```python
from build123d import *

# Parameters (mm, degrees)
SKETCH001_R  = 4.5
HOLE_DEPTH   = 25
POCKET_DEPTH = 10


with BuildPart() as part:
    # Sketch → Revolution (revolve)
    with BuildSketch(Plane.XZ):
        Polygon((0, 0), (0, 15), (5.15, 15), (5.15, 4), (7, 4), (7, 0), align=None)
    revolve(axis=Axis((0, 0, 0), (0, 0, 1)))

    # Sketch001 (on Face1 of Revolution) → Hole (cut)
    with BuildSketch(Plane(origin=(0, 0, 15), x_dir=(-1, 0, 0), z_dir=(0, 0, 1))):
        Circle(SKETCH001_R)
    extrude(amount=-HOLE_DEPTH, mode=Mode.SUBTRACT)

    # Sketch002 → Pocket (cut, symmetric)
    with BuildSketch(Plane.XZ):
        Polygon((-1.9, 15), (-1.9, 11), (-5.15, 11), (-5.15, 15), (-5.15, 18.504541), (5.249575, 18.504541), (5.249575, 15), (5.249575, 11), (1.9, 11), (1.9, 15), align=None)
    extrude(amount=POCKET_DEPTH, both=True, mode=Mode.SUBTRACT)


solid = part.part
```
CAD build for the part. Positions are in the model's coordinates, mm. A direction names the side the tool comes from. Round coordinates to 2 decimals unless told otherwise and drop trailing zeros. Order: outer loops, then holes, each group sorted by start corner. A loop starts at its lowest first (then second) coordinate and runs counter-clockwise, first axis right, second up.
Q1. Which spindle directions (+Z, -Z, +X, -X, +Y, -Y) get a long thin tool onto all of the face, cutting with end or side? Do faces 4 (the flat face through (4, 4, 4)), 5 (the flat face through (0, 5, 15)), 6 (the flat face through (5, 0, 11)), 7 (the flat face through (-5, 0, 11)). Say none if no direction does.
Q2. Two-plate mould, pull along X, no slides. Class faces 1 (the flat face through (0, -5, 15)), 2 (the cylindrical face through (4.496, -0.198, 5.938)), 3 (the cylindrical face through (-5.145, 0.226, 8.201)): pulls with the +X half, pulls with the -X half, needs draft (parallel to the pull), parting line crosses it, or undercut.
Q3. Drop flat-ended pins along their axis: pin 1 (1 mm diameter, centred on x = 4, y = 0.5, fed in from +Z); pin 2 (0.6 mm diameter, centred on y = 4.5, z = 13, fed in from -X); pin 3 (6 mm diameter, centred on x = 5.5, y = -1, fed in from -Z); pin 4 (1.5 mm diameter, centred on x = 4, z = 8, fed in from -Y) (3 decimals). Give the stop position or say it passes through.
Q4. Slice it at A-A (z = 11.5). Write the cut outline in (x, y).
Q5. Wall check: L1, parallel to Y at x = 0, z = 9.25; L2, parallel to Y at x = 0, z = 3.5. Give the ranges that are in metal, low to high.
Q6. Slice it at B-B (y = 0). Write the cut outline in (x, z).
Q7. Slice it at D-D (z = 1.75). Write the cut outline in (x, y), and give its area (3 significant figures).
Q8. Slice it at C-C (x = 0). Write the cut outline in (y, z).
Results below:
1. face 4: +Z
1. face 5: +Z, +X, -X, +Y, -Y
1. face 6: +Z, +X, +Y, -Y
1. face 7: +Z, -X, +Y, -Y
2. face 1: needs draft
2. face 2: undercut
2. face 3: parting line crosses it
3. pin 1: stops at z = 11
3. pin 2: stops at x = -1.9
3. pin 3: stops at z = 0
3. pin 4: stops at y = -3.995
4. outline: (-1.9, -4.79) arc R5.15 ccw to (1.9, -4.79) - (1.9, -4.08) arc R4.5 cw to (-1.9, -4.08) - close; (-1.9, 4.08) arc R4.5 cw to (1.9, 4.08) - (1.9, 4.79) arc R5.15 ccw to (-1.9, 4.79) - close
5. L1: y = -5.15 to -4.5, 4.5 to 5.15
5. L2: y = -7 to -4.5, 4.5 to 7
6. outline: (-7, 0) - (-4.5, 0) - (-4.5, 11) - (-5.15, 11) - (-5.15, 4) - (-7, 4) - close; (4.5, 0) - (7, 0) - (7, 4) - (5.15, 4) - (5.15, 11) - (4.5, 11) - close
7. outline: circle Ø14 at (0, 0); hole circle Ø9 at (0, 0)
7. area: 90.3 mm2
8. outline: (-7, 0) - (-4.5, 0) - (-4.5, 15) - (-5.15, 15) - (-5.15, 4) - (-7, 4) - close; (4.5, 0) - (7, 0) - (7, 4) - (5.15, 4) - (5.15, 15) - (4.5, 15) - close
